```python
from build123d import *

# Parameters (mm, degrees)
ESQUISSE1_W             = 42
ESQUISSE1_H             = 42
BOSS_EXTRU_1_DEPTH      = 8
CHANFREIN1_SIZE         = 5
ESQUISSE2_R             = 11
BOSS_EXTRU_2_DEPTH      = 2
ESQUISSE5_R             = 4.5
ENL_V_MAT_EXTRU_1_DEPTH = 3
CHANFREIN2_SIZE         = 0.3
BOSS_EXTRU_3_DEPTH      = 22
CONG_1_R                = 4
BOSS_EXTRU_4_DEPTH      = 9
ENL_V_START             = -3
ESQUISSE8_R             = 4.5
ENL_V_MAT_EXTRU_2_DEPTH = 3
TROU_TARAUD_M31_D       = 2.5
ESQUISSE9_R             = 2.5
ENL_V_MAT_EXTRU_3_DEPTH = 49.228622207


with BuildPart() as part:
    # Esquisse1 → Boss.-Extru.1 (new body)
    with BuildSketch(Plane(origin=(0, 0, 0), x_dir=(1, 0, 0), z_dir=(0, 1, 0))):
        Rectangle(ESQUISSE1_W, ESQUISSE1_H)
    extrude(amount=-BOSS_EXTRU_1_DEPTH)

    # Chanfrein1
    chanfrein1_edges = [part.edges().sort_by_distance(p)[0] for p in [
        (-21, -4, -21),
        (21, -4, -21),
        (21, -4, 21),
        (-21, -4, 21),
    ]]
    chamfer(chanfrein1_edges, length=CHANFREIN1_SIZE)

    # Esquisse2 → Boss.-Extru.2 (add)
    with BuildSketch(Plane(origin=(0, 0, 0), x_dir=(-1, 0, 0), z_dir=(0, -1, 0))):
        with Locations(Location((0, 0, 0), (0, 0, 90))):
            Circle(ESQUISSE2_R)
    extrude(amount=-BOSS_EXTRU_2_DEPTH)

    # Esquisse5 → Enlèv. mat.-Extru.1 (cut)
    with BuildSketch(Plane(origin=(0, 2, 0), x_dir=(1, 0, 0), z_dir=(0, 1, 0))):
        with Locations(Location((0, 0, 0), (0, 0, 270))):
            Circle(ESQUISSE5_R)
    extrude(amount=-ENL_V_MAT_EXTRU_1_DEPTH, mode=Mode.SUBTRACT)

    # Chanfrein2
    chanfrein2_edges = [part.edges().sort_by_distance(p)[0] for p in [
        (0, 0, 11),
        (0, 2, 11),
        (0, 2, -4.5),
    ]]
    chamfer(chanfrein2_edges, length=CHANFREIN2_SIZE)

    # Esquisse6 → Boss.-Extru.3 (add)
    with BuildSketch(Plane.XZ.offset(8)):
        with BuildLine():
            Line((20.9, -13.718236038), (20.9, 13.718236038))
            ThreePointArc((20.9, 13.718236038), (17.67766953, 17.67766953), (13.718236038, 20.9))
            Line((13.718236038, 20.9), (-13.718236038, 20.9))
            ThreePointArc((-13.718236038, 20.9), (-17.67766953, 17.67766953), (-20.9, 13.718236038))
            Line((-20.9, 13.718236038), (-20.9, -13.718236038))
            ThreePointArc((-20.9, -13.718236038), (-17.67766953, -17.67766953), (-13.718236038, -20.9))
            Line((-13.718236038, -20.9), (13.718236038, -20.9))
            ThreePointArc((13.718236038, -20.9), (17.67766953, -17.67766953), (20.9, -13.718236038))
        make_face()
    extrude(amount=BOSS_EXTRU_3_DEPTH)

    # Congé1
    cong_1_edges = [part.edges().sort_by_distance(p)[0] for p in [
        (13.718236038, -19, -20.9),
        (20.9, -19, -13.718236038),
        (20.9, -19, 13.718236038),
        (13.718236038, -19, 20.9),
        (-13.718236038, -19, 20.9),
        (-20.9, -19, 13.718236038),
        (-20.9, -19, -13.718236038),
        (-13.718236038, -19, -20.9),
    ]]
    fillet(cong_1_edges, radius=CONG_1_R)

    # Esquisse7 → Boss.-Extru.4 (add)
    with BuildSketch(Plane.XZ.offset(30)):
        Polygon((-16, -21), (16, -21), (21, -16), (21, 16), (16, 21), (-16, 21), (-21, 16), (-21, -16), align=None)
    extrude(amount=BOSS_EXTRU_4_DEPTH)

    # Esquisse8 → Enlèv. mat.-Extru.2 (cut)
    with BuildSketch(Plane.XZ.offset(39).offset(ENL_V_START)):
        with Locations(Location((0, 0, 0), (0, 0, 90))):
            Circle(ESQUISSE8_R)
    extrude(amount=ENL_V_MAT_EXTRU_2_DEPTH, mode=Mode.SUBTRACT)

    # Trou taraudé M31 (through all)
    with Locations(Plane(origin=(-18.160222152, 0, -3.642693465), x_dir=(-1, 0, 0), z_dir=(0, 1, 0))):
        with Locations((-33.716571339, 19.199042651), (-33.716571339, -11.913655721), (-2.603872966, -11.913655721), (-2.603872966, 19.199042651)):
            Hole(TROU_TARAUD_M31_D / 2)

    # Esquisse9 → Enlèv. mat.-Extru.3 (cut, through all)
    with BuildSketch(Plane(origin=(0, -1, 0), x_dir=(1, 0, 0), z_dir=(0, 1, 0))):
        with Locations(Location((0, 0, 0), (0, 0, 270))):
            Circle(ESQUISSE9_R)
    extrude(amount=-ENL_V_MAT_EXTRU_3_DEPTH, mode=Mode.SUBTRACT)


solid = part.part
```
Geometry: final body of the model. Coordinates: model frame, mm. A direction names the side the tool comes from. Round coordinates to 2 decimals unless told otherwise and drop trailing zeros. Write each loop counter-clockwise with the first axis right and the second up, starting at its lowest first coordinate (ties: lowest second). Pieces come first, ordered by that corner, then holes.
Item 1: Material intervals for L1, parallel to X at y = -17.5, z = 0; L2, parallel to X at y = -37, z = 0; L3, parallel to X at y = -6, z = -15, sorted ascending.
Item 2: Set-up query: faces 5 (the face through (-19, -30, -17)), 6 (the face through (-10.74, 0.99, 2.38)), 7 (the face through (20.9, -19, 0)), 8 (the face through (17.641, -18.846, -17.715)), 9 (the face through (-17.715, -18.846, -17.641)). Return all of +Z, -Z, +X, -X, +Y, -Y with unobstructed straight access to the full face (end or side cutting, diameter ignored); none if empty.
Item 3: Mould query, pull axis Y, two halves, no side actions, for faces 1 (the face through (0, -39, 5)), 2 (the face through (21, -4, 0)), 3 (the face through (9, 0, 9)), 4 (the face through (17.715, -18.846, 17.641)). Classes: +Y half, -Y half, draft (parallel to the pull), parting line (faces both ways), or undercut.
Item 4: Pin query (flat end, axial travel): P1, Ø3, axis at x = 0, z = 0, coming from the -Y side; P2, Ø5, axis at x = -11, z = 4.5, coming from the +Y side; P3, Ø10, axis at x = 11, z = 12.5, coming from the +Y side; P4, Ø6.5, axis at y = -18.5, z = -0.5, coming from the -X side. Return the tip coordinate at first contact, or that it passes through.
Item 5: Section query C-C (y = -26). Return loops of the section in (x, z), plus the area to 3 significant figures.
Completed:
1. L1: x = -20.9 to -2.5, 2.5 to 20.9
1. L2: x = -21 to -4.5, 4.5 to 21
1. L3: x = -21 to -16.68, -14.44 to 14.44, 16.68 to 21
2. face 5: none
2. face 6: +Y
2. face 7: +Z, -Z, +X
2. face 8: -Z, +X
2. face 9: -Z, -X
3. face 1: -Y half
3. face 2: draft
3. face 3: +Y half
3. face 4: undercut
4. P1: passes through
4. P2: stops at y = 2
4. P3: stops at y = 0
4. P4: stops at x = -20.9
5. outline: (-20.9, -12.47) arc R4 ccw to (-20.12, -14.84) arc R25 ccw to (-14.84, -20.12) arc R4 ccw to (-12.47, -20.9) - (12.47, -20.9) arc R4 ccw to (14.84, -20.12) arc R25 ccw to (20.12, -14.84) arc R4 ccw to (20.9, -12.47) - (20.9, 12.47) arc R4 ccw to (20.12, 14.84) arc R25 ccw to (14.84, 20.12) arc R4 ccw to (12.47, 20.9) - (-12.47, 20.9) arc R4 ccw to (-14.84, 20.12) arc R25 ccw to (-20.12, 14.84) arc R4 ccw to (-20.9, 12.47) - close; hole circle Ø2.5 at (-15.56, -15.56); hole circle Ø2.5 at (-15.56, 15.56); hole circle Ø5 at (0, 0); hole circle Ø2.5 at (15.56, -15.56); hole circle Ø2.5 at (15.56, 15.56)
5. area: 1,620 mm2
